Input: part model. Units: mm. Frame: model coordinates. Face numbers are marked on the shaded views. A direction names the side the tool comes from. Give positions to 0.01 mm unless a question says otherwise; leave off trailing zeros. Loops run counter-clockwise (first coordinate to the right, second up) from the corner with the lowest first, then second, coordinate; pieces in that order, holes last. Notation, with made-up numbers: (-18, 68.25) - (23, 68.25) arc R15 ccw to (23, 78.25) - close; hole circle Ø2 at (-33, 87). An arc over 180 degrees is marked (long way). Answer as a JSON object with one key per item and string values.
from build123d import *

# Parameters (mm, degrees)
MODEL_R                  = 2.0999999
STRUCTURAL_MEMBER1_DEPTH = 25


with BuildPart() as part:
    # Model → Structural Member1 (new body)
    with BuildSketch(Plane.ZX):
        with BuildLine():
            Line((-10, -13.3000005), (-10, -19))
            ThreePointArc((-10, -19), (-9.707106781, -19.707106781), (-9, -20))
            Line((-9, -20), (-3.3, -20))
            ThreePointArc((-3.3, -20), (-3.087867966, -19.912132034), (-3, -19.7))
            Line((-3, -19.7), (-3, -18))
            Line((-3, -18), (-6, -18))
            Line((-6, -18), (-6, -17.0606825))
            Line((-6, -17.0606825), (-2.939318, -14))
            Line((-2.939318, -14), (-0.519615242, -14))
            Line((-0.519615242, -14), (0, -13.7))
            Line((0, -13.7), (0.519615242, -14))
            Line((0.519615242, -14), (2.9393365, -14))
            Line((2.9393365, -14), (6, -17.0606628))
            Line((6, -17.0606628), (6, -18))
            Line((6, -18), (3, -18))
            Line((3, -18), (3, -19.7))
            ThreePointArc((3, -19.7), (3.087867966, -19.912132034), (3.3, -20))
            Line((3.3, -20), (9, -20))
            ThreePointArc((9, -20), (9.707106781, -19.707106781), (10, -19))
            Line((10, -19), (10, -13.3000005))
            ThreePointArc((10, -13.3000005), (9.912132034, -13.087868466), (9.7, -13.0000005))
            Line((9.7, -13.0000005), (8, -13.0000005))
            Line((8, -13.0000005), (8, -16.0000005))
            Line((8, -16.0000005), (7.06065685, -16.0000005))
            Line((7.06065685, -16.0000005), (4, -12.93934215))
            Line((4, -12.93934215), (4, -10.519615742))
            Line((4, -10.519615742), (3.7, -10.0000005))
            Line((3.7, -10.0000005), (4, -9.480385258))
            Line((4, -9.480385258), (4, -7.06068365))
            Line((4, -7.06068365), (7.06068236, -4.000000504))
            Line((7.06068236, -4.000000504), (8, -4.000000504))
            Line((8, -4.000000504), (8, -7.0000005))
            Line((8, -7.0000005), (9.7, -7.0000005))
            ThreePointArc((9.7, -7.0000005), (9.912132034, -6.912132534), (10, -6.7000005))
            Line((10, -6.7000005), (10, 6.7))
            ThreePointArc((10, 6.7), (9.912132034, 6.912132034), (9.7, 7))
            Line((9.7, 7), (8, 7))
            Line((8, 7), (8, 4))
            Line((8, 4), (7.060678, 4))
            Line((7.060678, 4), (4, 7.06068075))
            Line((4, 7.06068075), (4, 9.480384758))
            Line((4, 9.480384758), (3.7, 10))
            Line((3.7, 10), (4, 10.519615242))
            Line((4, 10.519615242), (4, 12.93933675))
            Line((4, 12.93933675), (7.060661, 16))
            Line((7.060661, 16), (8, 16))
            Line((8, 16), (8, 13))
            Line((8, 13), (9.7, 13))
            ThreePointArc((9.7, 13), (9.912132034, 13.087867966), (10, 13.3))
            Line((10, 13.3), (10, 19))
            ThreePointArc((10, 19), (9.707106781, 19.707106781), (9, 20))
            Line((9, 20), (3.3, 20))
            ThreePointArc((3.3, 20), (3.087867966, 19.912132034), (3, 19.7))
            Line((3, 19.7), (3, 18))
            Line((3, 18), (6, 18))
            Line((6, 18), (6, 17.06065975))
            Line((6, 17.06065975), (2.939354, 14))
            Line((2.939354, 14), (0.519638625, 14))
            Line((0.519638625, 14), (0, 13.6999865))
            Line((0, 13.6999865), (-0.519638625, 14))
            Line((-0.519638625, 14), (-2.939335, 14))
            Line((-2.939335, 14), (-6, 17.060678))
            Line((-6, 17.060678), (-6, 18))
            Line((-6, 18), (-3, 18))
            Line((-3, 18), (-3, 19.7))
            ThreePointArc((-3, 19.7), (-3.087867966, 19.912132034), (-3.3, 20))
            Line((-3.3, 20), (-9, 20))
            ThreePointArc((-9, 20), (-9.707106781, 19.707106781), (-10, 19))
            Line((-10, 19), (-10, 13.3))
            ThreePointArc((-10, 13.3), (-9.912132034, 13.087867966), (-9.7, 13))
            Line((-9.7, 13), (-8, 13))
            Line((-8, 13), (-8, 16))
            Line((-8, 16), (-7.060642, 16))
            Line((-7.060642, 16), (-4, 12.9393565))
            Line((-4, 12.9393565), (-4, 10.519615242))
            Line((-4, 10.519615242), (-3.7, 10))
            Line((-3.7, 10), (-4, 9.480384758))
            Line((-4, 9.480384758), (-4, 7.06066))
            Line((-4, 7.06066), (-7.060659, 4))
            Line((-7.060659, 4), (-8, 4))
            Line((-8, 4), (-8, 7))
            Line((-8, 7), (-9.7, 7))
            ThreePointArc((-9.7, 7), (-9.912132034, 6.912132034), (-10, 6.7))
            Line((-10, 6.7), (-10, -6.7000005))
            ThreePointArc((-10, -6.7000005), (-9.912132034, -6.912132534), (-9.7, -7.0000005))
            Line((-9.7, -7.0000005), (-8, -7.0000005))
            Line((-8, -7.0000005), (-8, -4.0000005))
            Line((-8, -4.0000005), (-7.06066257, -4.0000005))
            Line((-7.06066257, -4.0000005), (-4, -7.0606688))
            Line((-4, -7.0606688), (-4, -9.480385258))
            Line((-4, -9.480385258), (-3.7, -10.0000005))
            Line((-3.7, -10.0000005), (-4, -10.519615742))
            Line((-4, -10.519615742), (-4, -12.9393575))
            Line((-4, -12.9393575), (-7.0606365, -16.0000005))
            Line((-7.0606365, -16.0000005), (-8, -16.0000005))
            Line((-8, -16.0000005), (-8, -13.0000005))
            Line((-8, -13.0000005), (-9.7, -13.0000005))
            ThreePointArc((-9.7, -13.0000005), (-9.912132034, -13.087868466), (-10, -13.3000005))
        make_face()
        with Locations((0, 10)):
            Circle(MODEL_R, mode=Mode.SUBTRACT)
        with Locations((0, -10.0000005)):
            Circle(MODEL_R, mode=Mode.SUBTRACT)
        with BuildLine():
            Line((-8, 1.6999995), (-8, -1.70000025))
            ThreePointArc((-8, -1.70000025), (-7.912132034, -1.912132284), (-7.7, -2.00000025))
            Line((-7.7, -2.00000025), (-7.063604538, -2.00000025))
            ThreePointArc((-7.063604538, -2.00000025), (-6.948800316, -2.022823986), (-6.851481305, -2.087861995))
            Line((-6.851481305, -2.087861995), (-2.939335, -6))
            Line((-2.939335, -6), (2.93933195, -6))
            Line((2.93933195, -6), (6.851479294, -2.087861656))
            ThreePointArc((6.851479294, -2.087861656), (6.948799922, -2.022824212), (7.06360515, -2.00000025))
            Line((7.06360515, -2.00000025), (7.7, -2.00000025))
            ThreePointArc((7.7, -2.00000025), (7.912132034, -1.912132284), (8, -1.70000025))
            Line((8, -1.70000025), (8, 1.6999995))
            ThreePointArc((8, 1.6999995), (7.912132034, 1.912131534), (7.7, 1.9999995))
            Line((7.7, 1.9999995), (7.06359945, 1.9999995))
            ThreePointArc((7.06359945, 1.9999995), (6.9487942, 2.022823721), (6.851474147, 2.087862153))
            Line((6.851474147, 2.087862153), (2.9393355, 6))
            Line((2.9393355, 6), (-2.939339, 6))
            Line((-2.939339, 6), (-6.851476944, 2.087862556))
            ThreePointArc((-6.851476944, 2.087862556), (-6.948795311, 2.022823488), (-7.063599538, 1.9999995))
            Line((-7.063599538, 1.9999995), (-7.7, 1.9999995))
            ThreePointArc((-7.7, 1.9999995), (-7.912132034, 1.912131534), (-8, 1.6999995))
        make_face(mode=Mode.SUBTRACT)
    extrude(amount=STRUCTURAL_MEMBER1_DEPTH)


solid = part.part
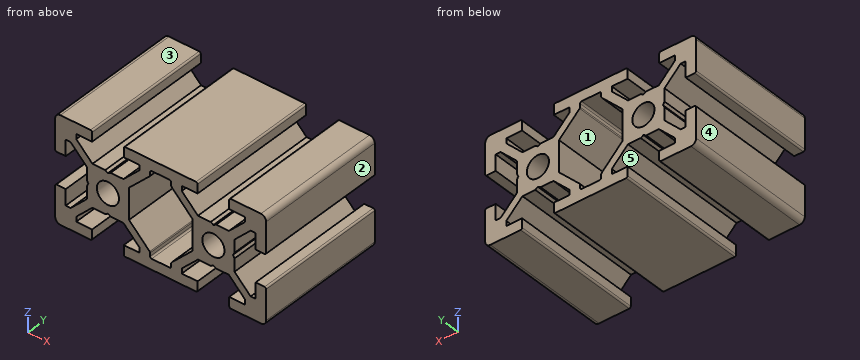
Item 1: Cut plane B-B (x = -2.5). Return loops of the section in (y, z).
Geometry check:
{"outline": "(0, -10) - (25, -10) - (25, -6.44) - (0, -6.44) - close; (0, 6.44) - (25, 6.44) - (25, 10) - (0, 10) - close"}
Item 2: Material intervals for line 1 (X direction, y = 10, z = 0); line 2 (X direction, y = 6.25, z = 8.5); line 3 (X direction, y = 7, z = 2.25), sorted ascending. Write a range as [from, to].
Geometry check:
{"line 1": "x = [-13.7, -12.1], [-7.9, -6], [6, 7.9], [12.1, 13.7]", "line 2": "x = [-20, -13], [-7, 7], [13, 20]", "line 3": "x = [-14, -6], [6, 14]"}
Item 3: Cut plane C-C (y = 18.25). Give the number of separate pieces and of enclosed holes in the cut face, then the cut area to 3 significant figures.
Geometry check:
{"separate pieces": "1", "enclosed holes": "3", "area": "324 mm2"}
Item 4: Cut plane D-D (x = 15). Return loops of the section in (y, z), then the cut area to 3 significant figures.
Geometry check:
{"outline": "(0, -10) - (25, -10) - (25, -8) - (0, -8) - close; (0, -6.06) - (25, -6.06) - (25, -3.94) - (0, -3.94) - close; (0, 3.94) - (25, 3.94) - (25, 6.06) - (0, 6.06) - close; (0, 8) - (25, 8) - (25, 10) - (0, 10) - close", "area": "206 mm2"}
Item 5: Access query for the marked faces 1 and 2. Directions: +Z, -Z, +X, -X, +Y, -Y. A direction counts if a zero-diameter tool reaches every point of the face in a straight line with its end or side. Return the directions, or none.
Geometry check:
{"face 1": "+Y, -Y", "face 2": "+Z, -Z, +X, +Y, -Y"}
Item 6: Cut plane A-A (z = 4.5). Return loops of the section in (x, y), then the cut area to 3 significant figures.
Geometry check:
{"outline": "(-20, 0) - (-18, 0) - (-18, 25) - (-20, 25) - close; (-15.56, 0) - (-13.44, 0) - (-13.44, 25) - (-15.56, 25) - close; (-6.56, 0) - (-4.44, 0) - (-4.44, 25) - (-6.56, 25) - close; (4.44, 0) - (6.56, 0) - (6.56, 25) - (4.44, 25) - close; (13.44, 0) - (15.56, 0) - (15.56, 25) - (13.44, 25) - close; (18, 0) - (20, 0) - (20, 25) - (18, 25) - close", "area": "312 mm2"}
Item 7: Mould query, pull axis X, two halves, no side actions, for the marked faces 3, 4 and 5. Classes: released by +X, released by -X, zero draft, split by the parting line, or undercut.
Geometry check:
{"face 3": "zero draft", "face 4": "released by -X", "face 5": "undercut"}
Item 8: Contact query for flat-ended pins moving along their axis: P1, Ø3.5, axis at x = 10, z = 0, coming from the -Y side; P2, Ø2, axis at x = 7, z = -2.5, coming from the -Y side; P3, Ø1, axis at x = -12, y = 14.5, coming from the +Z side; P4, Ø2.5, axis at x = 8.5, y = 13.5, coming from the -Z side. Output: stop coordinate, or through.
Geometry check:
{"P1": "passes through", "P2": "stops at y = 0", "P3": "stops at z = 4", "P4": "stops at z = -4"}
